Could you check a few things on this model? Use its own coordinates, in mm. Face numbers are marked on the shaded views. Give positions to 0.01 mm unless a question says otherwise; leave off trailing zeros. Order: outer loops, then holes, each group sorted by start corner. A loop starts at its lowest first (then second) coordinate and runs counter-clockwise, first axis right, second up. Notation, with made-up numbers: (46.25, 14.25) -> (70.25, 14.25) arc R21 cw to (70.25, 27.25) -> close; hole circle Ø4 at (7, 12). An arc over 180 degrees is marked (long way). Write each question's results on one line, items separated by ' | '.
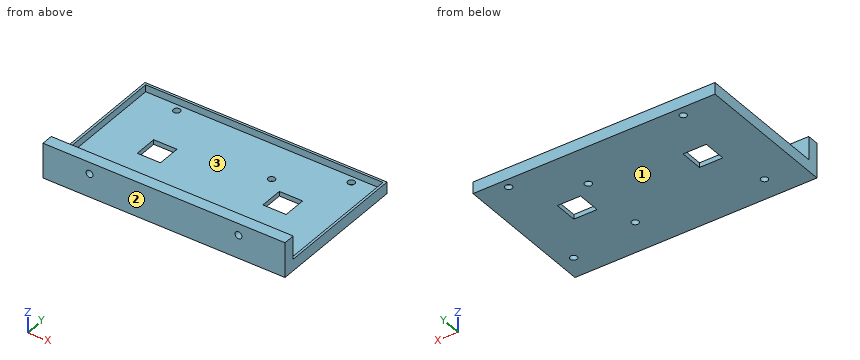
Autodesk Fusion 360 part; units mm, degrees
sketch "Esquisse2" plane through (0, 0, 0) normal (0, 0, 1) x (1, 0, 0)
  line L0 (0, 0) -> (104, 0)
  line L1 (104, 0) -> (104, 56)
  line L2 (104, 56) -> (0, 56)
  line L3 (0, 56) -> (0, 0)
  dimension "d1" = 104
  dimension "d2" = 56
extrude "Extrusion1" add sketch "Esquisse2" along normal blind 2
sketch "Esquisse3" plane through (0, 0, 2) normal (0, 0, 1) x (-1, 0, 0)
  line L0 (0, -56) -> (0, 0)
  line L1 (0, 0) -> (-104, 0)
  line L2 (-104, 0) -> (-104, -56)
  line L3 (-104, -56) -> (0, -56)
  line L4 (0, -56) -> (-104, -56)
  line L5 (-104, -56) -> (-104, 0)
  line L6 (-104, 0) -> (0, 0)
  line L7 (0, 0) -> (0, -56)
  line L8 (-1, -55) -> (-103, -55)
  line L9 (-103, -55) -> (-103, -1)
  line L10 (-103, -1) -> (-1, -1)
  line L11 (-1, -1) -> (-1, -55)
  dimension "d5" = 1
  dimension "d6" = 1
  dimension "d7" = 1
  dimension "d8" = 1
extrude "Extrusion2" add sketch "Esquisse3" along normal blind 3
sketch "Esquisse4" plane through (0, 0, 2) normal (0, 0, 1) x (-1, 0, 0)
  line L0 (-103, -1) -> (-103, -55)
  line L1 (-103, -55) -> (-1, -55)
  line L2 (-1, -55) -> (-1, -1)
  line L3 (-1, -1) -> (-103, -1)
  circle A0 centre (-16.5, -52) radius 1.5
  circle A1 centre (-15.5, -4) radius 1.5
  circle A2 centre (-67.5, -37.5) radius 1.5
  circle A3 centre (-67.5, -9) radius 1.5
  circle A4 centre (-91.5, -52) radius 1.5
  circle A5 centre (-97.5, -4) radius 1.5
  dimension "d11" = 3
  dimension "d12" = 3
  dimension "d13" = 3
  dimension "d14" = 3
  dimension "d15" = 3
  dimension "d16" = 3
  dimension "d17" = 3
  dimension "d18" = 15.5
  dimension "d19" = 3
  dimension "d20" = 14.5
  dimension "d21" = 35.5
  dimension "d22" = 17.5
  dimension "d23" = 35.5
  dimension "d24" = 8
  dimension "d25" = 11.5
  dimension "d26" = 3
  dimension "d27" = 3
  dimension "d28" = 5.5
extrude "Extrusion3" cut sketch "Esquisse4" against normal blind 5 contours A0 | A1 | A2 | A3 | A4 | A5
sketch "Esquisse6" plane through (0, 0, 0) normal (0, 0, -1) x (1, 0, 0)
  circle A0 centre (15.5, -4) radius 1.5
  circle A1 centre (91.5, -52) radius 1.5
  circle A2 centre (67.5, -9) radius 1.5
  circle A3 centre (16.5, -52) radius 1.5
  circle A4 centre (67.5, -37.5) radius 1.5
  circle A5 centre (97.5, -4) radius 1.5
  line L0 (0, 0) -> (0, -56)
  line L1 (0, -56) -> (104, -56)
  line L2 (104, -56) -> (104, 0)
  line L3 (104, 0) -> (0, 0)
  line L4 (20, -23) -> (30, -23)
  line L5 (30, -23) -> (30, -33)
  line L6 (30, -33) -> (20, -33)
  line L7 (20, -33) -> (20, -23)
  line L8 (74, -23) -> (84, -23)
  line L9 (84, -23) -> (84, -33)
  line L10 (84, -33) -> (74, -33)
  line L11 (74, -33) -> (74, -23)
  dimension "d34" = 10
  dimension "d35" = 10
  dimension "d36" = 10
  dimension "d37" = 10
  dimension "d38" = 20
  dimension "d39" = 23
  dimension "d40" = 23
  dimension "d41" = 20
extrude "Extrusion4" cut sketch "Esquisse6" against normal blind 5 contours L4 L5 L6 L7 | L8 L9 L10 L11
sketch "Esquisse7" plane through (0, 0, 0) normal (0, -1, 0) x (1, 0, 0)
  line L0 (0, 0) -> (104, 0)
  line L1 (104, 0) -> (104, 5)
  line L2 (104, 5) -> (0, 5)
  line L3 (0, 5) -> (0, 0)
  line L4 (0, 0) -> (104, 0)
  line L5 (104, 0) -> (104, 5)
  line L6 (104, 5) -> (0, 5)
  line L7 (0, 5) -> (0, 0)
extrude "Extrusion5" add sketch "Esquisse7" along normal blind 6
sketch "Esquisse8" plane through (0, 0, 5) normal (0, 0, 1) x (-1, 0, 0)
  line L0 (-103, -1) -> (-1, -1)
  line L1 (-1, -1) -> (-1, -55)
  line L2 (-1, -55) -> (-103, -55)
  line L3 (-103, -55) -> (-103, -1)
  line L4 (-104, 6) -> (-104, -56)
  line L5 (-104, -56) -> (0, -56)
  line L6 (0, -56) -> (0, 6)
  line L7 (0, 6) -> (-104, 6)
  line L8 (0, 6) -> (-104, 6)
  line L9 (-104, 6) -> (-104, 1)
  line L10 (-104, 1) -> (0, 1)
  line L11 (0, 1) -> (0, 6)
  dimension "d46" = 5
extrude "Extrusion6" add sketch "Esquisse8" along normal blind 10 contours L4 L6 L7 L8 L9 L10 L11
sketch "Esquisse9" plane through (0, -1, 0) normal (0, 1, 0) x (-1, 0, 0)
  line L0 (-104, 5) -> (0, 5)
  line L1 (0, 5) -> (0, 15)
  line L2 (0, 15) -> (-104, 15)
  line L3 (-104, 15) -> (-104, 5)
  circle A0 centre (-20, 10) radius 1.5
  circle A1 centre (-84, 10) radius 1.5
  dimension "d49" = 3
  dimension "d50" = 3
  dimension "d51" = 20
  dimension "d52" = 20
  dimension "d53" = 5
  dimension "d54" = 5
extrude "Extrusion7" cut sketch "Esquisse9" against normal blind 5 contours A0 | A1
Q1. Suppose I cut it at B-B on z = 10. Please give me the cut outline in (x, y), and give its area (3 significant figures).
Here are the results:
outline: (0, -6) -> (18.5, -6) -> (18.5, -1) -> (0, -1) -> close; (21.5, -6) -> (82.5, -6) -> (82.5, -1) -> (21.5, -1) -> close; (85.5, -6) -> (104, -6) -> (104, -1) -> (85.5, -1) -> close | area: 490 mm²
Q2. Suppose I cut it at A-A on y = 26. Please give me the cut outline in (x, z), and give its area (3 significant figures).
Here are the results:
outline: (0, 0) -> (20, 0) -> (20, 2) -> (1, 2) -> (1, 5) -> (0, 5) -> close; (30, 0) -> (74, 0) -> (74, 2) -> (30, 2) -> close; (84, 0) -> (104, 0) -> (104, 5) -> (103, 5) -> (103, 2) -> (84, 2) -> close | area: 174 mm²
Q3. Thinking about a two-plate mould opening in Y: for the marked faces 1, 2 and 3, which applies, +Y half, -Y half, draft (parallel to the pull), parting line (faces both ways), or undercut?
Here are the results:
face 1: draft | face 2: -Y half | face 3: undercut
Q4. I need wall thicknesses on line 1 along Y through (x, z) = (67.5, 1.3); line 2 along X through (y, z) = (52, 1.05); line 3 along Y through (x, z) = (59, 4.25). Which ranges of each line are inside material? Lowest first, please.
Here are the results:
line 1: y = -6 to 7.5, 10.5 to 36, 39 to 56 | line 2: x = 0 to 15, 18 to 90, 93 to 104 | line 3: y = -6 to 1, 55 to 56
Q5. I'm going to push flat-ended pins straight in: pin 1 Ø3 at (x, y) = (51.5, 49.5) entering from +Z; pin 2 Ø3 at (x, y) = (13.5, 1.5) entering from +Z. Where does each tip first touch, or does it pass through?
Here are the results:
pin 1: stops at z = 2 | pin 2: stops at z = 5
Q6. Suppose I cut it at D-D on z = 3. Please give me the cut outline in (x, y).
Here are the results:
outline: (0, -6) -> (104, -6) -> (104, 56) -> (0, 56) -> close; hole (1, 1) -> (103, 1) -> (103, 55) -> (1, 55) -> close
Q7. Suppose I cut it at C-C on x = 97.5. Please give me the cut outline in (y, z).
Here are the results:
outline: (-6, 0) -> (2.5, 0) -> (2.5, 2) -> (1, 2) -> (1, 5) -> (-1, 5) -> (-1, 15) -> (-6, 15) -> close; (5.5, 0) -> (56, 0) -> (56, 5) -> (55, 5) -> (55, 2) -> (5.5, 2) -> close
